Build history of the part. All positions in model axes, mm. Round coordinates to 2 decimals unless told otherwise and drop trailing zeros. Write each loop counter-clockwise with the first axis right and the second up, starting at its lowest first coordinate (ties: lowest second). Pieces come first, ordered by that corner, then holes. Notation, with made-up numbers: (-3.5, 49.5) - (3.5, 49.5) arc R24 cw to (3.5, 59.5) - close; hole circle Ø4 at (77, -5). An arc over 180 degrees is marked (long way). Answer as a JSON object with one key per item and string values. Group by question number.
Item 1: Slice it at B-B, the plane x = -21. List the corners of the cut face in (y, z), then the cut area to 3 significant figures.
Item 2: Flat gauge pins, fed straight in: pin 1 (4 mm diameter, centred on x = -59, z = 11, fed in from +Y); pin 2 (1.5 mm diameter, centred on x = -67.5, y = 13.5, fed in from -Z); pin 3 (10 mm diameter, centred on x = -47, y = 9.5, fed in from +Z); pin 4 (1.5 mm diameter, centred on y = 40.5, z = 11, fed in from -X). Where does each tip first touch, or does it go through?
Item 3: Two-plate mould, pull along Y, no slides. Class faces 1 (the cylindrical face through (-12.136, -15.616, 2.05)), 2 (the flat face through (0, -10.2, -6.2)), 3 (the cylindrical face through (-11.15, -3.529, -11.207)): +Y half, -Y half, draft (parallel to the pull), parting line (faces both ways), or undercut.
Item 4: Probe line 1 (Z direction, x = -15, y = 0); line 2 (X direction, y = 37.5, z = 1.5). List the from-to ranges inside material, lowest first. Write a range as from..to.
Item 5: Slice it at A-A, the plane z = 0. List the corners of the cut face in (x, y), then the cut area to 3 significant figures.
from build123d import *

# Parameters (mm, degrees)
ESQUISSE2_R     = 15.75
ESQUISSE2_R_2   = 11.75
CHANFREIN1_SIZE = 2


with BuildPart() as part:
    # Balayage2: sweep along a path in Esquisse1
    with BuildLine(Plane.XY) as balayage2_path:
        Line((0, 0), (-21.991698472, 0))
        ThreePointArc((-21.991698472, 0), (-44.934755926, 7.233918228), (-59.579403303, 26.319194267))
        Line((-59.579403303, 26.319194267), (-67.101007166, 46.984631039))
    # Esquisse2 → Balayage2 (sweep)
    with BuildSketch(Plane(origin=(0, 0, 0), x_dir=(0, 0, -1), z_dir=(1, 0, 0))):
        Circle(ESQUISSE2_R)
        Circle(ESQUISSE2_R_2, mode=Mode.SUBTRACT)
    sweep(path=balayage2_path.line)

    # Chanfrein1
    chanfrein1_edges = [part.edges().sort_by_distance(p)[0] for p in [
        (-67.101007166, 46.984631039, 15.75),
        (0, 0, 15.75),
    ]]
    chamfer(chanfrein1_edges, length=CHANFREIN1_SIZE)


solid = part.part
Geometry says:
{
 "1": {"outline": "circle Ø31.5 at (0, 0); hole circle Ø23.5 at (0, 0)", "area": "346 mm^2"},
 "2": {"pin 1": "stops at y = 50.4", "pin 2": "stops at z = -10.3", "pin 3": "stops at z = 15.75", "pin 4": "stops at x = -77.52"},
 "3": {"face 1": "parting line", "face 2": "draft", "face 3": "undercut"},
 "4": {"line 1": "z = -15.75..-11.75, 11.75..15.75", "line 2": "x = -80.33..-76.05, -51.25..-46.96"},
 "5": {"outline": "(-81.22, 39.72) - (-74.38, 20.93) arc R55.75 ccw to (-21.99, -15.75) - (-2, -15.75) - (0, -13.75) - (0, -11.75) - (-21.99, -11.75) arc R51.75 cw to (-70.62, 22.3) - (-78.14, 42.97) - (-80.02, 42.28) - close; (-56.06, 51) - (-48.54, 30.34) arc R28.25 ccw to (-21.99, 11.75) - (0, 11.75) - (0, 13.75) - (-2, 15.75) - (-21.99, 15.75) arc R24.25 cw to (-44.78, 31.71) - (-51.62, 50.49) - (-54.18, 51.69) - close", "area": "735 mm^2"}
}
